Work out the finished part from the listing and answer in its coordinate system (mm). Face numbers are marked on the shaded views. A direction names the side the tool comes from. Round coordinates to 2 decimals unless told otherwise and drop trailing zeros. Write each loop counter-clockwise with the first axis right and the second up, starting at its lowest first coordinate (ties: lowest second). Pieces come first, ordered by that corner, then holes. Notation, with made-up numbers: (75.5, 73.5) - (88.5, 73.5) arc R23 ccw to (88.5, 94.5) - close; hole circle Ø8 at (8, 42). An arc over 180 degrees is marked (long way). Answer as a JSON object with one key per item and string values.
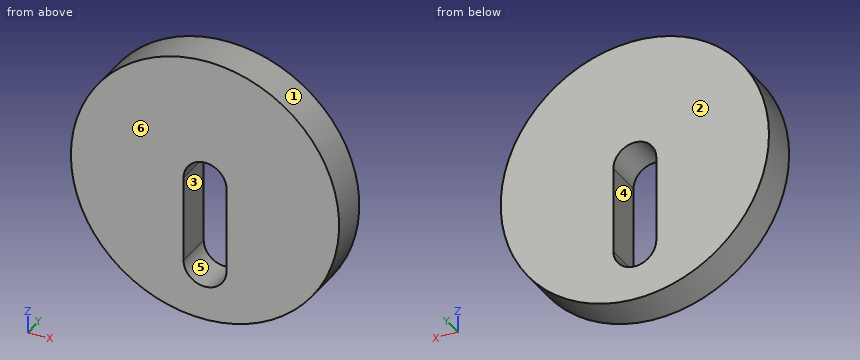
Autodesk Inventor part; units mm, degrees
ref_plane "YZ Plane" through (0, 0, 0) normal (1, 0, 0) x (0, 1, 0)
ref_plane "XZ Plane" through (0, 0, 0) normal (0, 1, 0) x (-1, 0, 0)
ref_plane "XY Plane" through (0, 0, 0) normal (0, 0, 1) x (1, 0, 0)
sketch "スケッチ1" plane through (0, 0, 0) normal (0, 1, 0) x (-1, 0, 0)
  circle A0 centre (0, 0) radius 22.5 construction
  circle A1 centre (0, 0) radius 25.5 construction
  line L0 (25.5, 1.2181) -> (25.5, -1.2181)
  line L1 (25.5, 1.2181) -> (22.3764, 2.355)
  line L2 (25.5, -1.2181) -> (22.3764, -2.355)
  line L3 (35.7, 0) -> (-35.7, 0)
  circle A2 centre (0, 0) radius 18.75
  line L4 (22.3764, -2.355) -> (18.647, -1.9625)
  line L5 (22.3764, 2.355) -> (18.647, 1.9625)
  line L6 (19.484, 11.2527) -> (16.2367, 9.3773)
  line L7 (22.8, 11.4846) -> (19.484, 11.2527)
  line L8 (22.8, 11.4846) -> (23.7909, 9.259)
  line L9 (23.7909, 9.259) -> (21.3997, 6.9499)
  line L10 (21.3997, 6.9499) -> (17.8331, 5.7916)
  line L11 (13.2226, 18.2047) -> (11.0189, 15.1706)
  line L12 (16.1576, 19.7653) -> (13.2226, 18.2047)
  line L13 (16.1576, 19.7653) -> (17.9681, 18.1351)
  line L14 (17.9681, 18.1351) -> (16.7229, 15.0531)
  line L15 (16.7229, 15.0531) -> (13.9357, 12.5443)
  line L16 (4.675, 22.009) -> (3.8958, 18.3408)
  line L17 (6.7214, 24.6284) -> (4.675, 22.009)
  line L18 (6.7214, 24.6284) -> (9.0384, 23.8755)
  line L19 (9.0384, 23.8755) -> (9.1544, 20.5535)
  line L20 (9.1544, 20.5535) -> (7.6287, 17.1279)
  line L21 (-4.6811, 22.0077) -> (-3.9009, 18.3397)
  line L22 (-3.8769, 25.233) -> (-4.6811, 22.0077)
  line L23 (-3.8769, 25.233) -> (-1.454, 25.4876)
  line L24 (-1.454, 25.4876) -> (0.0031, 22.5)
  line L25 (0.0031, 22.5) -> (0.0026, 18.75)
  line L26 (-13.2277, 18.201) -> (-11.0231, 15.1675)
  line L27 (-13.8049, 21.4746) -> (-13.2277, 18.201)
  line L28 (-13.8049, 21.4746) -> (-11.6951, 22.6927)
  line L29 (-11.6951, 22.6927) -> (-9.1487, 20.556)
  line L30 (-9.1487, 20.556) -> (-7.6239, 17.13)
  line L31 (-19.4871, 11.2473) -> (-16.2393, 9.3727)
  line L32 (-21.3459, 14.0031) -> (-19.4871, 11.2473)
  line L33 (-21.3459, 14.0031) -> (-19.9139, 15.974)
  line L34 (-19.9139, 15.974) -> (-16.7187, 15.0578)
  line L35 (-16.7187, 15.0578) -> (-13.9322, 12.5481)
  line L36 (-22.3771, 2.3488) -> (-18.6476, 1.9573)
  line L37 (-25.196, 4.1103) -> (-22.3771, 2.3488)
  line L38 (-25.196, 4.1103) -> (-24.6895, 6.4932)
  line L39 (-24.6895, 6.4932) -> (-21.3978, 6.9559)
  line L40 (-21.3978, 6.9559) -> (-17.8315, 5.7965)
  line L41 (-21.3978, -6.9559) -> (-17.8315, -5.7965)
  line L42 (-24.6895, -6.4932) -> (-21.3978, -6.9559)
  line L43 (-24.6895, -6.4932) -> (-25.196, -4.1103)
  line L44 (-25.196, -4.1103) -> (-22.3771, -2.3488)
  line L45 (-22.3771, -2.3488) -> (-18.6476, -1.9573)
  line L46 (-16.7187, -15.0578) -> (-13.9322, -12.5481)
  line L47 (-19.9139, -15.974) -> (-16.7187, -15.0578)
  line L48 (-19.9139, -15.974) -> (-21.3459, -14.0031)
  line L49 (-21.3459, -14.0031) -> (-19.4871, -11.2473)
  line L50 (-19.4871, -11.2473) -> (-16.2393, -9.3727)
  line L51 (-9.1487, -20.556) -> (-7.6239, -17.13)
  line L52 (-11.6951, -22.6927) -> (-9.1487, -20.556)
  line L53 (-11.6951, -22.6927) -> (-13.8049, -21.4746)
  line L54 (-13.8049, -21.4746) -> (-13.2277, -18.201)
  line L55 (-13.2277, -18.201) -> (-11.0231, -15.1675)
  line L56 (0.0031, -22.5) -> (0.0026, -18.75)
  line L57 (-1.454, -25.4876) -> (0.0031, -22.5)
  line L58 (-1.454, -25.4876) -> (-3.8769, -25.233)
  line L59 (-3.8769, -25.233) -> (-4.6811, -22.0077)
  line L60 (-4.6811, -22.0077) -> (-3.9009, -18.3397)
  line L61 (9.1544, -20.5535) -> (7.6287, -17.1279)
  line L62 (9.0384, -23.8755) -> (9.1544, -20.5535)
  line L63 (9.0384, -23.8755) -> (6.7214, -24.6284)
  line L64 (6.7214, -24.6284) -> (4.675, -22.009)
  line L65 (4.675, -22.009) -> (3.8958, -18.3408)
  line L66 (16.7229, -15.0531) -> (13.9357, -12.5443)
  line L67 (17.9681, -18.1351) -> (16.7229, -15.0531)
  line L68 (17.9681, -18.1351) -> (16.1576, -19.7653)
  line L69 (16.1576, -19.7653) -> (13.2226, -18.2047)
  line L70 (13.2226, -18.2047) -> (11.0189, -15.1706)
  line L71 (21.3997, -6.9499) -> (17.8331, -5.7916)
  line L72 (23.7909, -9.259) -> (21.3997, -6.9499)
  line L73 (23.7909, -9.259) -> (22.8, -11.4846)
  line L74 (22.8, -11.4846) -> (19.484, -11.2527)
  line L75 (19.484, -11.2527) -> (16.2367, -9.3773)
  circle A3 centre (0, 0) radius 11
  point P0 (25.5, 0)
  point P1 (23.2954, 10.3718)
  point P2 (17.0628, 18.9502)
  point P3 (7.8799, 24.2519)
  point P4 (-2.6655, 25.3603)
  point P5 (-12.75, 22.0836)
  point P6 (-20.6299, 14.9885)
  point P7 (-24.9428, 5.3017)
  point P8 (-24.9428, -5.3017)
  point P9 (-20.6299, -14.9885)
  point P10 (-12.75, -22.0836)
  point P11 (-2.6655, -25.3603)
  point P12 (7.8799, -24.2519)
  point P13 (17.0628, -18.9502)
  point P14 (23.2954, -10.3718)
  point P15 (17.8331, 5.7916)
  point P16 (16.2367, 9.3773)
  point P17 (13.9357, 12.5443)
  point P18 (11.0189, 15.1706)
  point P19 (7.6287, 17.1279)
  point P20 (3.8958, 18.3408)
  point P21 (0.0026, 18.75)
  point P22 (-3.9009, 18.3397)
  point P23 (-7.6239, 17.13)
  point P24 (-11.0231, 15.1675)
  point P25 (-13.9322, 12.5481)
  point P26 (-16.2393, 9.3727)
  point P27 (-17.8315, 5.7965)
  point P28 (-18.6476, 1.9573)
  point P29 (-18.6476, -1.9573)
  point P30 (-17.8315, -5.7965)
  point P31 (-16.2393, -9.3727)
  point P32 (-13.9322, -12.5481)
  point P33 (-11.0231, -15.1675)
  point P34 (-7.6239, -17.13)
  point P35 (-3.9009, -18.3397)
  point P36 (0.0026, -18.75)
  point P37 (3.8958, -18.3408)
  point P38 (7.6287, -17.1279)
  point P39 (11.0189, -15.1706)
  point P40 (13.9357, -12.5443)
  point P41 (16.2367, -9.3773)
  point P42 (17.8331, -5.7916)
  dimension "d5" = 37.5
  dimension "d0" = 45
  dimension "d1" = 51
  dimension "d3" = 20
  dimension "d4" = 20
  dimension "d14" = 4.71
  dimension "d18" = 360
  dimension "d23" = 22
extrude "押し出し1" add sketch "スケッチ1" along normal blind 5.5 contours A2 L3 A3 | L3 A3 A2 | A3 L3 | L3 A3
sketch "スケッチ2" plane through (0, 5.5, 0) normal (0, 1, 0) x (1, 0, 0)
  circle A0 centre (0, 10) radius 3 construction
  circle A1 centre (0, 0) radius 3 construction
  line L0 (-3, 10) -> (-3, 0)
  line L1 (3, 10) -> (3, 0)
  circle A2 centre (0, 11) radius 3
  circle A3 centre (0, -1) radius 3
  line L2 (3, 10) -> (3, 11)
  line L3 (-3, 10) -> (-3, 11)
  line L4 (3, 0) -> (3, -1)
  line L5 (-3, 0) -> (-3, -1)
  dimension "d30" = 6
  dimension "d31" = 6
  dimension "d32" = 10
  dimension "d33" = 6
  dimension "d34" = 6
  dimension "d35" = 1
  dimension "d36" = 1
extrude "押し出し2" cut sketch "スケッチ2" against normal through all
properties part number "M3_15_ホーン" material "木材 (カエデ材)"
Item 1: A cutting plane is placed at C-C (y = 4.45). Write down the section's boundary in (x, z).
Results found:
{"outline": "circle Ø37.5 at (0, 0); hole (-3, -11) arc R3 ccw to (3, -11) - (3, 1) arc R3 ccw to (-3, 1) - close"}
Item 2: Determine the mould class of the marked faces 1, 2, 3 and 4 for opening direction X: pulls with the +X half, pulls with the -X half, needs draft (parallel to the pull), parting line crosses it, or undercut.
Results found:
{"face 1": "parting line crosses it", "face 2": "needs draft", "face 3": "undercut", "face 4": "undercut"}
Item 3: A cutting plane is placed at B-B (z = 0). Write down the section's boundary in (x, y), and give its area (3 significant figures).
Results found:
{"outline": "(-18.75, 0) - (-3, 0) - (-3, 5.5) - (-18.75, 5.5) - close; (3, 0) - (18.75, 0) - (18.75, 5.5) - (3, 5.5) - close", "area": "173 mm²"}
Item 4: A cutting plane is placed at A-A (x = 0). Write down the section's boundary in (y, z), and give its area (3 significant figures).
Results found:
{"outline": "(0, -18.75) - (5.5, -18.75) - (5.5, -14) - (0, -14) - close; (0, 4) - (5.5, 4) - (5.5, 18.75) - (0, 18.75) - close", "area": "107 mm²"}
Item 5: A cutting plane is placed at D-D (z = 8). Write down the section's boundary in (x, y).
Results found:
{"outline": "(-16.96, 0) - (16.96, 0) - (16.96, 5.5) - (-16.96, 5.5) - close"}
Item 6: Consider line 1 along X through (y, z) = (1.45, 0); line 2 along X through (y, z) = (0.6, -7.5); line 3 along X through (y, z) = (0.4, 11). Determine where each line is inside the solid, lowest interval first.
Results found:
{"line 1": "-18.75 to -3, 3 to 18.75", "line 2": "-17.18 to -3, 3 to 17.18", "line 3": "-15.18 to 15.18"}
Item 7: For the marked faces 5 and 6, determine the directions among +Z, -Z, +X, -X, +Y, -Y from which every point of the face is accessible in a straight line to the end or side of a thin tool.
Results found:
{"face 5": "+Y, -Y", "face 6": "+Z, -Z, +X, -X, -Y"}
Item 8: Each of these flat-tipped pins is pushed along its axis until it touches: P1, Ø2, axis at x = 12.5, z = -3.5, coming from the -Y side; P2, Ø3, axis at y = 1.5, z = -2.5, coming from the -X side; P3, Ø1, axis at x = -10, y = 2.5, coming from the +Z side; P4, Ø1.6, axis at y = 2.5, z = -2.5, coming from the +X side. Where does it stop, or does it pass through?
Results found:
{"P1": "y = 0", "P2": "x = -18.72", "P3": "z = 16.17", "P4": "x = 18.67"}
